Part print with two shaded views. Sizes in mm from the minimum x, y, z corner. Round coordinates to 2 decimals unless told otherwise and drop trailing zeros. Loops run counter-clockwise (first coordinate to the right, second up) from the corner with the lowest first, then second, coordinate; pieces in that order, holes last.
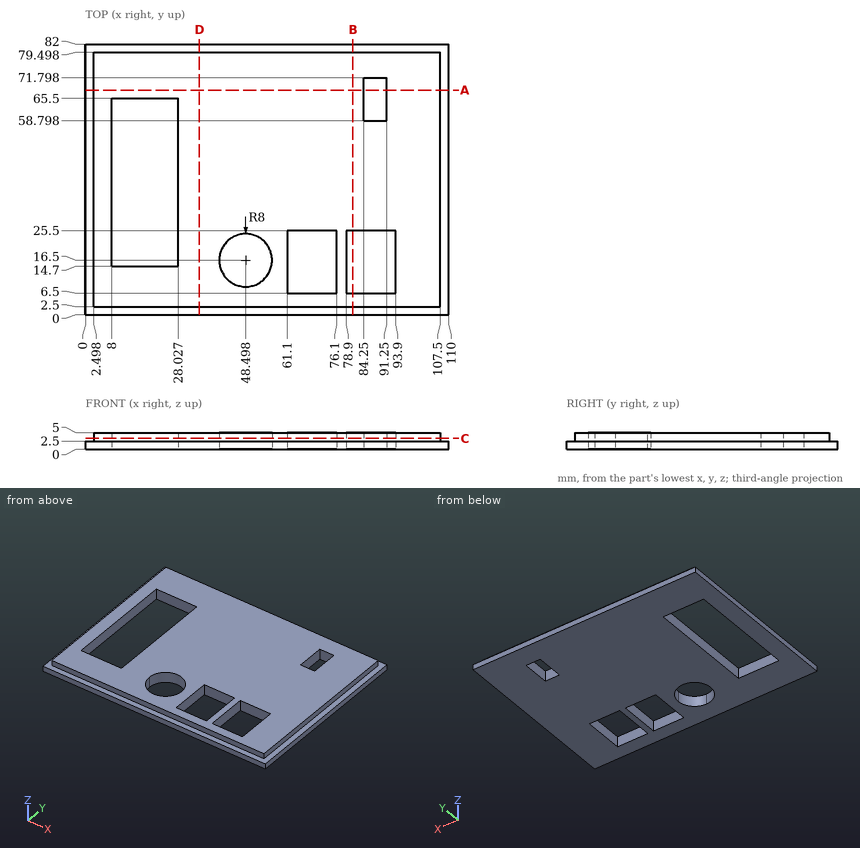
Item 1: Cut at C-C (z = 3.3). List the corners of the cut face in (x, y).
Verdict:
outline: (2.5, 2.5) - (107.5, 2.5) - (107.5, 79.5) - (2.5, 79.5) - close; hole (8, 14.7) - (28.03, 14.7) - (28.03, 65.5) - (8, 65.5) - close; hole circle Ø16 at (48.5, 16.5); hole (61.1, 6.5) - (76.1, 6.5) - (76.1, 25.5) - (61.1, 25.5) - close; hole (78.9, 6.5) - (93.9, 6.5) - (93.9, 25.5) - (78.9, 25.5) - close; hole (84.25, 58.8) - (91.25, 58.8) - (91.25, 71.8) - (84.25, 71.8) - close
Item 2: Flat gauge pin, fed straight in: P1, Ø3, axis at x = 56.5, z = 4.5, coming from the -Y side. Where does the tip first touch, or does it go through?
Verdict:
P1: stops at y = 2.5
Item 3: Cut at B-B (x = 81). List the corners of the cut face in (y, z).
Verdict:
outline: (0, 0) - (6.5, 0) - (6.5, 5) - (2.5, 5) - (2.5, 2.5) - (0, 2.5) - close; (25.5, 0) - (82, 0) - (82, 2.5) - (79.5, 2.5) - (79.5, 5) - (25.5, 5) - close
Item 4: Cut at A-A (y = 68). List the corners of the cut face in (x, z).
Verdict:
outline: (0, 0) - (84.25, 0) - (84.25, 5) - (2.5, 5) - (2.5, 2.5) - (0, 2.5) - close; (91.25, 0) - (110, 0) - (110, 2.5) - (107.5, 2.5) - (107.5, 5) - (91.25, 5) - close
Item 5: Cut at D-D (x = 34.5). List the corners of the cut face in (y, z).
Verdict:
outline: (0, 0) - (82, 0) - (82, 2.5) - (79.5, 2.5) - (79.5, 5) - (2.5, 5) - (2.5, 2.5) - (0, 2.5) - close
Item 6: Wall check: L1, parallel to Y at x = 90, z = 3.2; L2, parallel to X at y = 63, z = 2.9; L3, parallel to X at y = 12, z = 2.2 (1 decimal). Give the ranges that are in metal, low to high.
Verdict:
L1: y = 2.5 to 6.5, 25.5 to 58.8, 71.8 to 79.5
L2: x = 2.5 to 8, 28.03 to 84.25, 91.25 to 107.5
L3: x = 0 to 41.9, 55.1 to 61.1, 76.1 to 78.9, 93.9 to 110
